The listing builds one solid part. Answer for the finished solid, in the listing's coordinates (mm). Coordinates: 2 decimals unless noted, no trailing zeros. Write each loop counter-clockwise with the first axis right and the second up, starting at its lowest first coordinate (ties: lowest second). Pieces come first, ordered by that corner, then holes.
Autodesk Inventor part; units mm, degrees
ref_plane "YZ Plane" through (0, 0, 0) normal (1, 0, 0) x (0, 1, 0)
ref_plane "XZ Plane" through (0, 0, 0) normal (0, 1, 0) x (-1, 0, 0)
ref_plane "XY Plane" through (0, 0, 0) normal (0, 0, 1) x (1, 0, 0)
sketch "Эскиз1" plane through (0, 0, 0) normal (1, 0, 0) x (0, 1, 0)
  line L0 (0, 19) -> (10, 19)
  line L1 (10, 19) -> (10, -19)
  line L2 (10, -19) -> (0, -19)
  line L3 (0, -19) -> (0, 19)
  line L4 (-2, 0) -> (12, 0) construction
  line L5 (0, -26.6) -> (0, 26.6) construction
  point P0 (0, 0)
  dimension "d0" = 10
  dimension "d1" = 38
extrude "Выдавливание1" add sketch "Эскиз1" along normal blind 46
sketch "Эскиз2" plane through (46, 0, 0) normal (1, 0, 0) x (0, 0, -1)
  line L0 (19, 10) -> (-19, 10)
  line L1 (-19, 10) -> (-19, 0)
  line L2 (19, 0) -> (19, 10)
  line L3 (0, -2) -> (0, 12) construction
  point P0 (0, 0)
  point P1 (-14, 5)
  point P2 (14, 5)
  dimension "d4" = 5
  dimension "d5" = 5
  dimension "d6" = 5
hole "Отверстие1" at (46, 5, 14) at (46, 5, -14) direction (-1, 0, 0) diameter 3 depth 60
chamfer "Фаска1" distance 0.2 angle 45 4 edges at (46, 5, -12.5) (46, 5, 15.5) (0, 5, -12.5) (0, 5, 15.5)
properties part number "Стенкка для ковнейера"
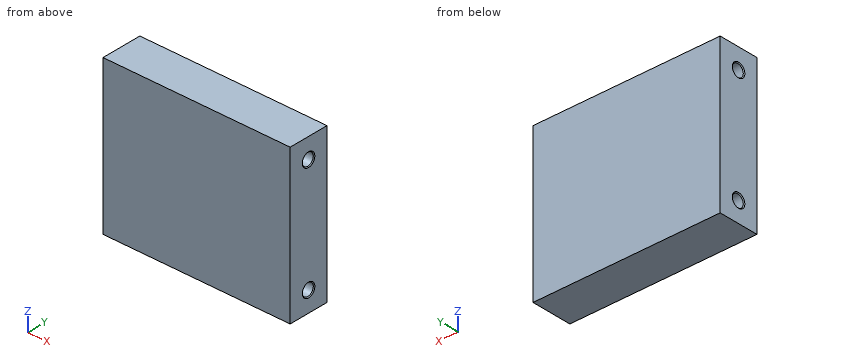
(1) This flat-tipped pin is pushed along its axis until it touches: pin 1 (4 mm diameter, centred on y = 5, z = 14, fed in from -X). Where does it stop, or does it pass through?
(2) Section B-B, the plane z = 14 is taken. Write down the section's boundary in (x, y), plus the area to 3 significant figures.
(3) Section C-C, the plane x = 23 is taken. Write down the section's boundary in (y, z), plus the area to 3 significant figures.
(4) Find the intervals of material crossed by probe 1 along Z at (x, y) = (32.5, 5); probe 2 along Y at (x, z) = (25, 14); probe 3 along Z at (x, y) = (33, 6), in increasing order.
(5) Section A-A, the plane y = 5 is taken. Write down the section's boundary in (x, z).
Solution:
1. pin 1: stops at x = 0
2. outline: (0, 0) - (46, 0) - (46, 3.3) - (45.8, 3.5) - (0.2, 3.5) - (0, 3.3) - close; (0, 6.7) - (0.2, 6.5) - (45.8, 6.5) - (46, 6.7) - (46, 10) - (0, 10) - close
2. area: 322 mm2
3. outline: (0, -19) - (10, -19) - (10, 19) - (0, 19) - close; hole circle Ø3 at (5, -14); hole circle Ø3 at (5, 14)
3. area: 366 mm2
4. probe 1: z = -19 to -15.5, -12.5 to 12.5, 15.5 to 19
4. probe 2: y = 0 to 3.5, 6.5 to 10
4. probe 3: z = -19 to -15.12, -12.88 to 12.88, 15.12 to 19
5. outline: (0, -19) - (46, -19) - (46, -15.7) - (45.8, -15.5) - (0.2, -15.5) - (0, -15.7) - close; (0, -12.3) - (0.2, -12.5) - (45.8, -12.5) - (46, -12.3) - (46, 12.3) - (45.8, 12.5) - (0.2, 12.5) - (0, 12.3) - close; (0, 15.7) - (0.2, 15.5) - (45.8, 15.5) - (46, 15.7) - (46, 19) - (0, 19) - close
